```python
from build123d import *

# Parameters (mm, degrees)
SKETCH1_R               = 2.413
BOSS_EXTRUDE1_DEPTH     = 847.09
SKETCH2_R               = 1.27
SKETCH2_R_2             = 0.28089526
CUT_EXTRUDE1_DEPTH      = 3.413
CUT_EXTRUDE1_DEPTH_BACK = 3.413


with BuildPart() as part:
    # Sketch1 → Boss-Extrude1 (new body)
    with BuildSketch(Plane.XY):
        Circle(SKETCH1_R)
    extrude(amount=BOSS_EXTRUDE1_DEPTH)

    # Sketch2 → Cut-Extrude1 (cut, two sides)
    with BuildSketch(Plane(origin=(0, 0, 0), x_dir=(1, 0, 0), z_dir=(0, 1, 0))) as cut_extrude1_sk:
        with Locations((0, -843.555959397)):
            Circle(SKETCH2_R)
        with Locations((0, -0.735765283)):
            Circle(SKETCH2_R_2)
    extrude(amount=CUT_EXTRUDE1_DEPTH, mode=Mode.SUBTRACT)
    extrude(cut_extrude1_sk.sketch, amount=-CUT_EXTRUDE1_DEPTH_BACK, mode=Mode.SUBTRACT)


solid = part.part
```
Part model, mm, in its own coordinate system. Round coordinates to 2 decimals unless told otherwise and drop trailing zeros. Write each loop counter-clockwise with the first axis right and the second up, starting at its lowest first coordinate (ties: lowest second). Pieces come first, ordered by that corner, then holes.
Item 1: Probe L1, parallel to Z at x = 0, y = 1.3; L2, parallel to Z at x = -0.2, y = 0.6; L3, parallel to Z at x = 0.4, y = 0.8. List the from-to ranges inside material, lowest first.
Results:
L1: z = 0 to 0.45, 1.02 to 842.29, 844.83 to 847.09
L2: z = 0 to 0.54, 0.93 to 842.3, 844.81 to 847.09
L3: z = 0 to 842.35, 844.76 to 847.09
Item 2: Cut at B-B, the plane z = 93. Give the cut face in (x, y), plus the area to 3 significant figures.
Results:
outline: circle Ø4.83 at (0, 0)
area: 18.3 mm2
Item 3: Cut at A-A, the plane y = -0.95. Give the cut face in (x, z), plus the area to 3 significant figures.
Results:
outline: (-2.22, 0) - (2.22, 0) - (2.22, 847.09) - (-2.22, 847.09) - close; hole circle Ø2.54 at (0, 843.56); hole circle Ø0.56 at (0, 0.74)
area: 3,750 mm2
Item 4: Drop a flat-ended pin along its axis: pin 1 Ø1 at (y, z) = (2, 587.5) entering from +X. Give the stop position or say it passes through.
Results:
pin 1: stops at x = 1.89
